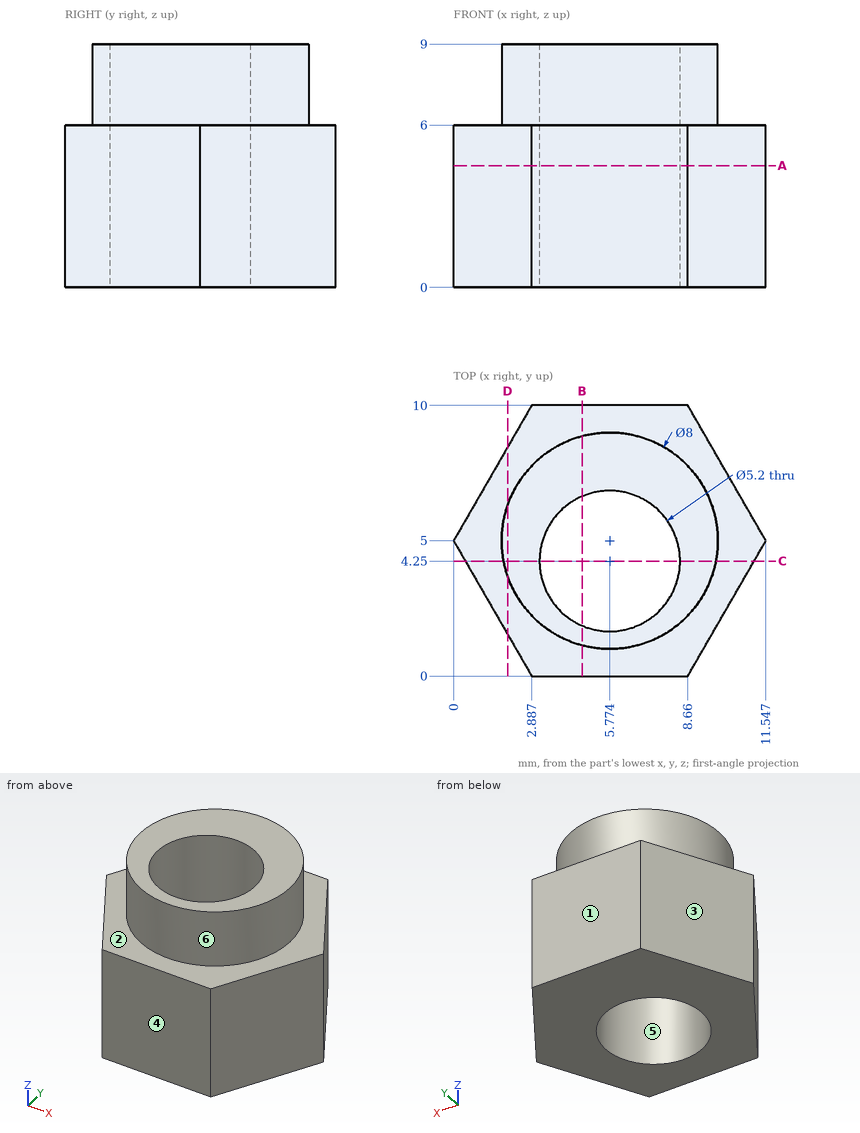
Study the drawing (mm; zero at the part's minimum x, y, z) and answer. A direction names the side the tool comes from. Coordinates: 2 decimals unless noted, no trailing zeros. Write each loop counter-clockwise with the first axis right and the second up, starting at its lowest first coordinate (ties: lowest second). Pieces come first, ordered by that corner, then holes. Notation, with made-up numbers: (-28.75, -10.75) - (12.25, -10.75) arc R34 cw to (12.25, 24.25) - close; hole circle Ø9 at (87.5, 67.25). An arc over 180 degrees is marked (long way). Answer as a JSON object with one key per item and string values. Group by question number.
1. Each of these flat-tipped pins is pushed along its axis until it touches: P1, Ø3, axis at x = 5.77, y = 4.25, coming from the -Z side; P2, Ø4, axis at x = 10, y = 2.5, coming from the -Z side; P3, Ø1.5, axis at y = 8, z = 5.5, coming from the +X side. Where does it stop, or does it pass through?
2. A cutting plane is placed at A-A (z = 4.5). Determine the outline of the cut face in (x, y).
3. A cutting plane is placed at C-C (y = 4.25). Determine the outline of the cut face in (x, z) (1 decimal).
4. A cutting plane is placed at B-B (x = 4.75). Determine the outline of the cut face in (y, z).
5. Consider L1, parallel to Y at x = 6.5, z = 1.25 (1 decimal); L2, parallel to Z at x = 3, y = 8.75; L3, parallel to Y at x = 8, z = 1.75 (1 decimal). Determine where each line is inside the solid, lowest interval first. Write a range as [from, to].
6. A cutting plane is placed at D-D (x = 2). Determine the outline of the cut face in (y, z) (1 decimal).
7. Which of the six approach directions +Z, -Z, +X, -X, +Y, -Y give full straight-line access (tool end or side, diameter ignored) to the marked faces 1 and 2?
8. The mould has two halves that part along X. Classify the marked faces 3, 4, 5 and 6: +X half, -X half, draft (parallel to the pull), parting line (faces both ways), or undercut.
Worked out:
{
 "1": {"P1": "passes through", "P2": "stops at z = 0", "P3": "stops at x = 10.25"},
 "2": {"outline": "(0, 5) - (2.89, 0) - (8.66, 0) - (11.55, 5) - (8.66, 10) - (2.89, 10) - close; hole circle Ø5.2 at (5.77, 4.25)"},
 "3": {"outline": "(0.4, 0) - (3.2, 0) - (3.2, 9) - (1.8, 9) - (1.8, 6) - (0.4, 6) - close; (8.4, 0) - (11.1, 0) - (11.1, 6) - (9.7, 6) - (9.7, 9) - (8.4, 9) - close"},
 "4": {"outline": "(0, 0) - (1.86, 0) - (1.86, 9) - (1.13, 9) - (1.13, 6) - (0, 6) - close; (6.64, 0) - (10, 0) - (10, 6) - (8.87, 6) - (8.87, 9) - (6.64, 9) - close"},
 "5": {"L1": "y = [0, 1.8], [6.7, 10]", "L2": "z = [0, 6]", "L3": "y = [0, 2.9], [5.6, 10]"},
 "6": {"outline": "(1.5, 0) - (8.5, 0) - (8.5, 6) - (6.3, 6) - (6.3, 9) - (3.7, 9) - (3.7, 6) - (1.5, 6) - close"},
 "7": {"face 1": "+Z, -Z, +X, -X, +Y", "face 2": "+Z"},
 "8": {"face 3": "-X half", "face 4": "draft", "face 5": "undercut", "face 6": "parting line"}
}
